Geometry: see drawing. Coordinates: mm, zero at the bounding-box minimum. A direction names the side the tool comes from. Coordinates: 2 decimals unless noted, no trailing zeros. Order: outer loops, then holes, each group sorted by start corner. A loop starts at its lowest first (then second) coordinate and runs counter-clockwise, first axis right, second up.
Item 1: Section B-B on x = 7.5. Return the cut outline in (y, z).
Item 2: Section A-A on y = 7.9. Return the cut outline in (x, z), then the cut area to 3 significant figures.
Item 3: Ray query, line 1 (X direction, y = 12, z = 4.75); line 2 (Y direction, x = 6, z = 2.25); line 3 (Y direction, x = 8.5, z = 11.5). Return the intervals inside material, ascending.
Item 4: Contact query for flat-ended pins moving along their axis: P1, Ø7, axis at y = 9, z = 4.5, coming from the +X side; P2, Ø2, axis at y = 12.5, z = 3, coming from the +X side; P3, Ø4, axis at y = 4, z = 4.5, coming from the -X side; P4, Ø5, axis at y = 11.5, z = 10.5, coming from the +X side. Output: stop coordinate, or through.
Item 5: Reachability of the marked faces 1 and 2 from +Z, -Z, +X, -X, +Y, -Y: full face, straight path, thin tool, end or side. Return the list, or none.
Item 6: Section C-C on z = 10.75. Return the cut outline in (x, y).
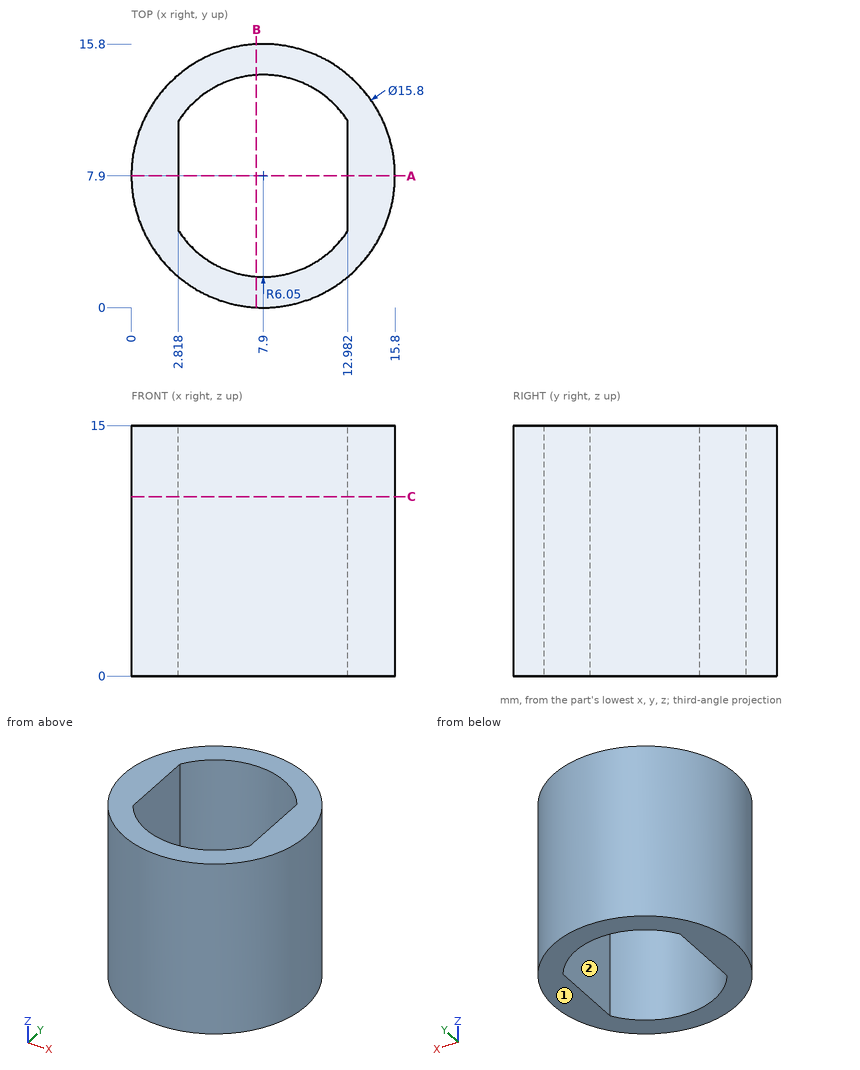
Answer list:
1. outline: (0.01, 0) - (1.86, 0) - (1.86, 15) - (0.01, 15) - close; (13.94, 0) - (15.79, 0) - (15.79, 15) - (13.94, 15) - close
2. outline: (0, 0) - (2.82, 0) - (2.82, 15) - (0, 15) - close; (12.98, 0) - (15.8, 0) - (15.8, 15) - (12.98, 15) - close
2. area: 84.5 mm2
3. line 1: x = 1.15 to 3.45, 12.35 to 14.65
3. line 2: y = 0.23 to 2.16, 13.64 to 15.57
3. line 3: y = 0.02 to 1.88, 13.92 to 15.78
4. P1: stops at x = 15.8
4. P2: stops at x = 14.93
4. P3: stops at x = 0.23
4. P4: stops at x = 15.72
5. face 1: -Z, +X, -X, +Y, -Y
5. face 2: +Z, -Z
6. outline: circle Ø15.8 at (7.9, 7.9); hole (2.82, 4.62) arc R6.05 ccw to (12.98, 4.62) - (12.98, 11.18) arc R6.05 ccw to (2.82, 11.18) - close
